Build history of the part. All positions in model axes, mm. A direction names the side the tool comes from. Give positions to 0.01 mm unless a question says otherwise; leave off trailing zeros. Write each loop counter-clockwise with the first axis right and the second up, starting at its lowest first coordinate (ties: lowest second). Pieces come first, ordered by that corner, then holes. Notation, with made-up numbers: (6, 63.25) -> (45, 63.25) arc R26 ccw to (45, 84.25) -> close; hole circle Ø8 at (-20.75, 88.25). An arc over 180 degrees is marked (long way). Write item = value, one per line. Start each with the question number.
Q1. Drop flat-ended pins along their axis: P1, Ø1.5, axis at x = -6, y = 5, coming from the -Z side; P2, Ø1.6, axis at x = -9.5, z = -1, coming from the +Y side; P3, Ø3, axis at x = -0.5, y = 6, coming from the +Z side. Give the stop position or say it passes through.
Q2. Saw through at D-D, the plane x = 2. List the corners of the cut face in (y, z).
Q3. Saw through at B-B, the plane y = 4.75. List the corners of the cut face in (x, z).
Q4. Saw through at C-C, the plane z = 5.25. List the corners of the cut face in (x, y).
Q5. Saw through at A-A, the plane z = 15. List the corners of the cut face in (x, y) (3 decimals).
Q6. Mould opens along Z. For faces 5 (the face through (-1.838, 10.314, 11.875)), 6 (the face through (9, 8.2, -1)), 7 (the face through (1.787, 10.314, 11.846)), 8 (the face through (-9, 4, -1.5)) say: pulls with the +Z half, pulls with the -Z half, needs draft (parallel to the pull), parting line crosses it, or undercut.
Q7. Wall check: line 1 (X direction, y = 4.25, z = 15.5); line 2 (X direction, y = 12.4, z = 15); line 3 (Z direction, x = -0.25, y = -4.5). Give the ranges that are in metal, low to high.
Q8. Tool access for faces 1 (the face through (9, 0, -1)), 2 (the face through (-8.25, 4, -1)), 3 (the face through (0, 9.1, 20.3)), 4 (the face through (2.5, 11.7, 14.1)): list every direction of +Z, -Z, +X, -X, +Y, -Y with a clear straight run to the whole face (end or side of a thin tool).
from build123d import *

# Parameters (mm, degrees)
PAD_DEPTH       = 10
SKETCH001_W     = 14.1
SKETCH001_H     = 13.7
POCKET_DEPTH    = 14
SKETCH002_R     = 2.5
POCKET001_DEPTH = 23.501
SKETCH003_W     = 8.2
SKETCH003_H     = 16.5
POCKET002_DEPTH = 1.5
SKETCH004_R     = 2.5
POCKET003_DEPTH = 20.001
SKETCH005_R     = 5
POCKET004_DEPTH = 18
POCKET005_DEPTH = 3.5


with BuildPart() as part:
    # Sketch → Pad (new body, symmetric)
    with BuildSketch(Plane.YZ):
        Polygon((0, -1.5), (8.2, -1.5), (8.2, 0), (14.1, 0), (14.1, 22), (8.2, 22), (-5.9, 8), (-5.9, 0), (0, 0), align=None)
    extrude(amount=PAD_DEPTH, both=True)

    # Sketch001 (on Face8 of Pad) → Pocket (cut)
    with BuildSketch(Plane(origin=(0, 0, 22), x_dir=(0, -1, 0), z_dir=(0, 0, 1))):
        with Locations((-1.15, 0)):
            Rectangle(SKETCH001_W, SKETCH001_H)
    extrude(amount=-POCKET_DEPTH, mode=Mode.SUBTRACT)

    # Sketch002 (on Face11 of Pocket) → Pocket001 (cut, through all)
    with BuildSketch(Plane.YX.offset(1.5)):
        with Locations((4.1, 0)):
            Circle(SKETCH002_R)
    extrude(amount=-POCKET001_DEPTH, mode=Mode.SUBTRACT)

    # Sketch003 (on Face11 of Pocket001) → Pocket002 (cut)
    with BuildSketch(Plane.YX.offset(1.5)):
        with Locations((4.1, 0)):
            Rectangle(SKETCH003_W, SKETCH003_H)
    extrude(amount=-POCKET002_DEPTH, mode=Mode.SUBTRACT)

    # Sketch004 (on Face14 of Pocket002) → Pocket003 (cut, through all)
    with BuildSketch(Plane.ZX.offset(14.1)):
        with Locations((15, 0)):
            Circle(SKETCH004_R)
    extrude(amount=-POCKET003_DEPTH, mode=Mode.SUBTRACT)

    # Sketch005 (on Face8 of Pocket003) → Pocket004 (cut)
    with BuildSketch(Plane(origin=(0, 0, 22), x_dir=(0, -1, 0), z_dir=(0, 0, 1))):
        with Locations((-4.1, 0)):
            Circle(SKETCH005_R)
    extrude(amount=-POCKET004_DEPTH, mode=Mode.SUBTRACT)

    # Sketch006 (on Face17 of Pocket004) → Pocket005 (cut)
    with BuildSketch(Plane(origin=(0, 8.2, 0), x_dir=(0, 0, -1), z_dir=(0, -1, 0))):
        Polygon((-10.814211, 0), (-12.907105, 3.625), (-17.092895, 3.625), (-19.185789, 0), (-17.092895, -3.625), (-12.907105, -3.625), align=None)
    extrude(amount=-POCKET005_DEPTH, mode=Mode.SUBTRACT)


solid = part.part
Report:
q1.P1 = 0
q1.P2 = 8.2
q1.P3 = 4
q2.outline = (-5.9, 0) -> (2.6, 0) -> (2.6, 4) -> (-0.48, 4) -> (-0.48, 8) -> (-5.9, 8) -> close; (5.6, 0) -> (14.1, 0) -> (14.1, 13.5) -> (11.7, 13.5) -> (11.7, 11.97) -> (8.68, 11.97) -> (8.68, 4) -> (5.6, 4) -> close; (8.68, 18.03) -> (11.7, 18.03) -> (11.7, 16.5) -> (14.1, 16.5) -> (14.1, 22) -> (8.68, 22) -> close
q3.outline = (-10, -1.5) -> (-8.25, -1.5) -> (-8.25, 0) -> (-2.41, 0) -> (-2.41, 4) -> (-4.96, 4) -> (-4.96, 8) -> (-6.85, 8) -> (-6.85, 18.57) -> (-10, 18.57) -> close; (2.41, 0) -> (8.25, 0) -> (8.25, -1.5) -> (10, -1.5) -> (10, 18.57) -> (6.85, 18.57) -> (6.85, 8) -> (4.96, 8) -> (4.96, 4) -> (2.41, 4) -> close
q4.outline = (-10, -5.9) -> (10, -5.9) -> (10, 14.1) -> (-10, 14.1) -> close; hole circle Ø10 at (0, 4.1)
q5.outline = (-10, 1.15) -> (-6.85, 1.15) -> (-6.85, 8.2) -> (-3.625, 8.2) -> (-3.625, 11.7) -> (-2.5, 11.7) -> (-2.5, 14.1) -> (-10, 14.1) -> close; (2.5, 11.7) -> (3.625, 11.7) -> (3.625, 8.2) -> (6.85, 8.2) -> (6.85, 1.15) -> (10, 1.15) -> (10, 14.1) -> (2.5, 14.1) -> close
q6.face_5 = undercut
q6.face_6 = needs draft
q6.face_7 = undercut
q6.face_8 = pulls with the -Z half
q7.line_1 = -10 to -6.85, 6.85 to 10
q7.line_2 = -10 to -2.5, 2.5 to 10
q7.line_3 = 0 to 8
q8.face_1 = -Z, +X, -X, -Y
q8.face_2 = -Z, +Y, -Y
q8.face_3 = +Z, -Y
q8.face_4 = -Y
